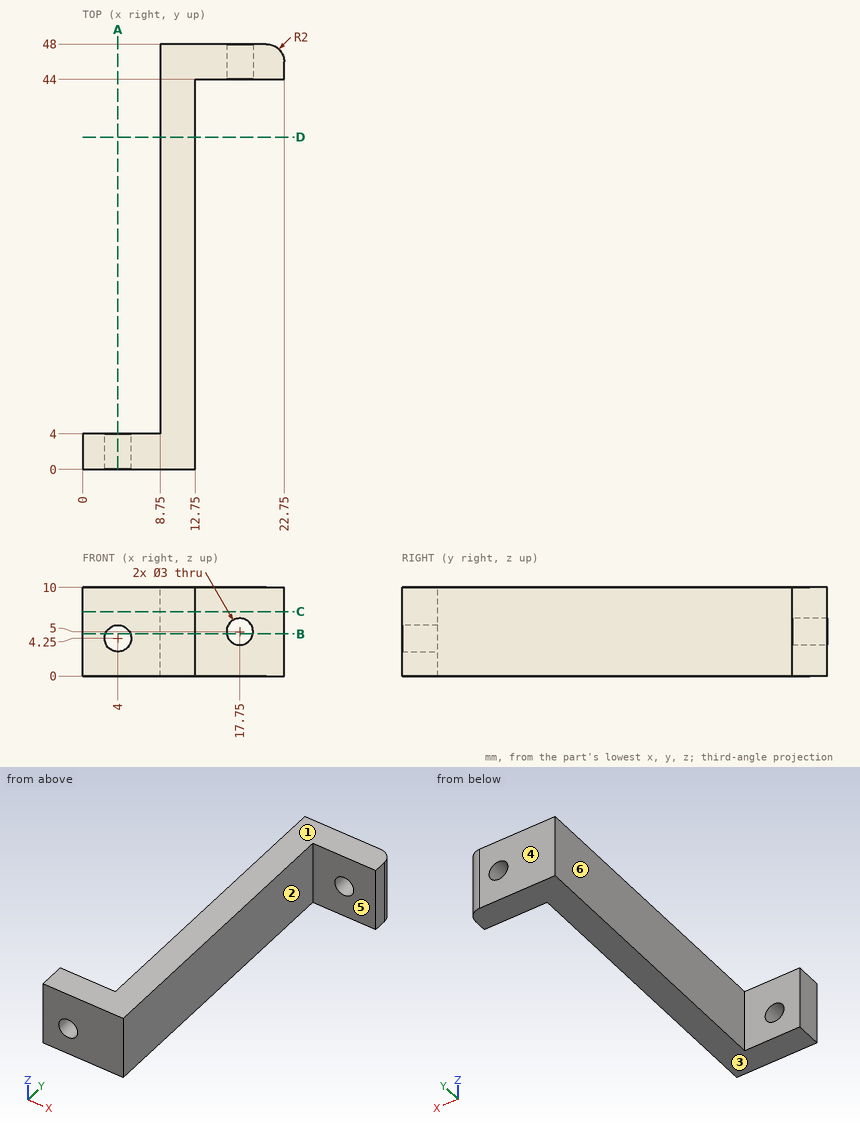
Here's the drawing with two shaded views (mm, measured from the low corner). I have some questions. A direction names the side the tool comes from. Coordinates: 2 decimals unless noted, no trailing zeros. Write each loop counter-clockwise with the first axis right and the second up, starting at its lowest first coordinate (ties: lowest second). Pieces come first, ordered by that corner, then holes. Notation, with made-up numbers: M 34.5,33.25 L 76.5,33.25 A19 ccw 76.5,37.25 Z; hole C 29.25,50.5 d10. An arc over 180 degrees is marked long. Answer as CSV lines item,"result". Start each with the question number.
1) I want a section at A-A, the plane x = 4. Please give me the cut outline in (y, z).
2) I want a section at C-C, the plane z = 7.25. Please give me the cut outline in (x, y), and give its area (3 significant figures).
3) We'd pull the mould along Z, two halves only. Please class the marked faces 1, 2 and 3: +Z half, -Z half, draft (parallel to the pull), parting line (faces both ways), or undercut.
4) For the marked faces 4, 5 and 6, which set-ups out of +Z, -Z, +X, -X, +Y, -Y let a thin tool reach every point of the face, with its end or its side?
5) For P1, Ø10, axis at x = 18, y = 16.5, coming from the +Z side; P2, Ø3, axis at y = 21, z = 4.5, coming from the -X side; P3, Ø1.5, axis at y = 28, z = 2.5, coming from the +X side; P4, Ø1, axis at x = 2.5, z = 9, coming from the +Y side, each with a flat end and sliding along its axis, tell me the tip position at first contact or that it passes through.
6) I want a section at D-D, the plane y = 37.5. Please give me the cut outline in (x, z).
7) I want a section at B-B, the plane z = 4.75. Please give me the cut outline in (x, y).
8) Please list where these lines run through material, in increasing order: line 1 (X direction, y = 3, z = 4.25); line 2 (Y direction, x = 7.25, z = 3); line 3 (X direction, y = 42, z = 4.25). Write a range as from..to.
Data:
1,outline,"M 0,0 L 4,0 L 4,2.75 L 0,2.75 Z; M 0,5.75 L 4,5.75 L 4,10 L 0,10 Z"
2,outline,"M 0,0 L 12.75,0 L 12.75,44 L 22.75,44 L 22.75,46 A2 ccw 20.75,48 L 8.75,48 L 8.75,4 L 0,4 Z"
2,area,"266 mm^2"
3,face 1,"+Z half"
3,face 2,"draft"
3,face 3,"-Z half"
4,face 4,"+Z, -Z, +X, -X, +Y"
4,face 5,"+Z, -Z, +X, -Y"
4,face 6,"+Z, -Z, -X, +Y"
5,P1,"passes through"
5,P2,"stops at x = 8.75"
5,P3,"stops at x = 12.75"
5,P4,"stops at y = 4"
6,outline,"M 8.75,0 L 12.75,0 L 12.75,10 L 8.75,10 Z"
7,outline,"M 0,0 L 2.59,0 L 2.59,4 L 0,4 Z; M 5.41,0 L 12.75,0 L 12.75,44 L 16.27,44 L 16.27,48 L 8.75,48 L 8.75,4 L 5.41,4 Z; M 19.23,44 L 22.75,44 L 22.75,46 A2 ccw 20.75,48 L 19.23,48 Z"
8,line 1,"x = 0..2.5, 5.5..12.75"
8,line 2,"y = 0..4"
8,line 3,"x = 8.75..12.75"
